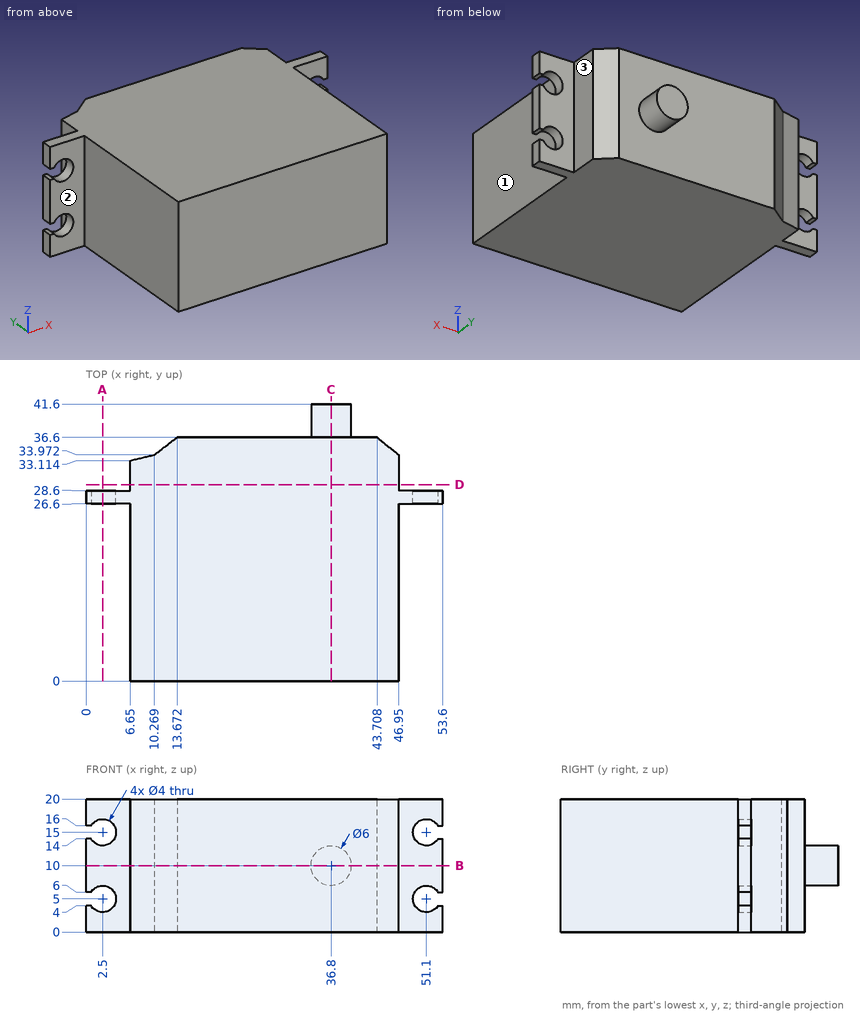
For this review, use the dimensioned drawing (mm, ordinates from the lowest corner) and the shaded views. A direction names the side the tool comes from. Coordinates: 2 decimals unless noted, no trailing zeros. Loops run counter-clockwise (first coordinate to the right, second up) from the corner with the lowest first, then second, coordinate; pieces in that order, holes last. Notation, with made-up numbers: (15.25, 29.25) -> (58.25, 29.25) arc R21 ccw to (58.25, 53.25) -> close; hole circle Ø3 at (81.5, 80). An arc over 180 degrees is marked (long way). Return JSON: item names as keys, results as strings. Group by question number.
(1) Consider section D-D, the plane y = 29.5. Give the boundary of the cut face in (x, z).
(2) Consider section A-A, the plane x = 2.5. Give the boundary of the cut face in (y, z), plus the area to 3 significant figures.
(3) Consider section C-C, the plane x = 36.8. Give the boundary of the cut face in (y, z), plus the area to 3 significant figures.
(4) To check wall thickness, follow L1, parallel to Z at x = 51.1, y = 27; L2, parallel to Z at x = 2, y = 27; L3, parallel to X at y = 25, z = 3. State the ranges of each line that lie inside material, in increasing order.
(5) Tool access review of the marked faces 1, 2 and 3: name each direction out of +Z, -Z, +X, -X, +Y, -Y from which nothing blocks a thin tool from reaching the whole face with its end or side.
(6) Consider section B-B, the plane z = 10. Give the boundary of the cut face in (x, y), plus the area to 3 significant figures.
(7) For pin 1 Ø1 at (y, z) = (5.5, 2.5) entering from +X; pin 2 Ø3.5 at (x, z) = (2.5, 5) entering from +Y; pin 3 Ø3.5 at (x, z) = (49, 10.5) entering from +Y; pin 4 Ø12 at (x, z) = (26, 13.5) entering from +Y, all flat-tipped, find the tip position at first contact; note any pin that passes through.
Results below:
{
 "1": {"outline": "(6.65, 0) -> (46.95, 0) -> (46.95, 20) -> (6.65, 20) -> close"},
 "2": {"outline": "(26.6, 0) -> (28.6, 0) -> (28.6, 3) -> (26.6, 3) -> close; (26.6, 7) -> (28.6, 7) -> (28.6, 13) -> (26.6, 13) -> close; (26.6, 17) -> (28.6, 17) -> (28.6, 20) -> (26.6, 20) -> close", "area": "24.0 mm2"},
 "3": {"outline": "(0, 0) -> (36.6, 0) -> (36.6, 7) -> (41.6, 7) -> (41.6, 13) -> (36.6, 13) -> (36.6, 20) -> (0, 20) -> close", "area": "762 mm2"},
 "4": {"L1": "z = 0 to 3, 7 to 13, 17 to 20", "L2": "z = 0 to 3.06, 6.94 to 13.06, 16.94 to 20", "L3": "x = 6.65 to 46.95"},
 "5": {"face 1": "+Z, -Z, +X, -Y", "face 2": "+Z, -Z, -X, -Y", "face 3": "+Z, -Z, +X, +Y"},
 "6": {"outline": "(0, 26.6) -> (6.65, 26.6) -> (6.65, 0) -> (46.95, 0) -> (46.95, 26.6) -> (53.6, 26.6) -> (53.6, 28.6) -> (46.95, 28.6) -> (46.95, 33.97) -> (43.71, 36.6) -> (39.8, 36.6) -> (39.8, 41.6) -> (33.8, 41.6) -> (33.8, 36.6) -> (13.67, 36.6) -> (10.27, 33.97) -> (6.65, 33.11) -> (6.65, 28.6) -> (0, 28.6) -> close", "area": "1,510 mm2"},
 "7": {"pin 1": "stops at x = 46.95", "pin 2": "passes through", "pin 3": "stops at y = 28.6", "pin 4": "stops at y = 36.6"}
}
